The listing builds one solid part. Answer for the finished solid, in the listing's coordinates (mm). Coordinates: 2 decimals unless noted, no trailing zeros. Loops run counter-clockwise (first coordinate to the right, second up) from the corner with the lowest first, then second, coordinate; pieces in that order, holes last. Notation, with made-up numbers: (65, 80.25) -> (113, 80.25) arc R18 cw to (113, 112.25) -> close; hole circle Ø8 at (42.5, 20). An arc over 180 degrees is marked (long way). Answer in a Markdown table with one row per item.
```python
from build123d import *

# Parameters (mm, degrees)
SKETCH1_R           = 8
BOSS_EXTRUDE1_DEPTH = 3
CUT_EXTRUDE1_DEPTH  = 133.578278764
CUT_EXTRUDE8_DEPTH  = 10
FILLET2_R           = 5
FILLET3_R           = 5
FILLET4_R           = 5


with BuildPart() as part:
    # Sketch1 → Boss-Extrude1 (new body)
    with BuildSketch(Plane.XY):
        with BuildLine():
            Line((0, -12), (-120, -12))
            ThreePointArc((-120, -12), (-132, 0), (-120, 12))
            Line((-120, 12), (0, 12))
            ThreePointArc((0, 12), (12, 0), (0, -12))
        make_face()
        with Locations((-120, 0)):
            Circle(SKETCH1_R, mode=Mode.SUBTRACT)
        with Locations(Location((0, 0, 0), (0, 0, 180))):
            Circle(SKETCH1_R, mode=Mode.SUBTRACT)
    extrude(amount=BOSS_EXTRUDE1_DEPTH)

    # Sketch2 → Cut-Extrude1 (cut, through all)
    with BuildSketch(Plane.XY.offset(3)):
        with BuildLine():
            Line((-17.036725037, 6), (-20.036725037, 6))
            ThreePointArc((-20.036725037, 6), (-18.824439071, 9.116514898), (-17.130976336, 12))
            Line((-17.130976336, 12), (-13.5, 12))
            ThreePointArc((-13.5, 12), (-15.560298648, 9.172082969), (-17.036725037, 6))
        make_face()
        with BuildLine():
            Line((-102.963274963, 6), (-99.963274963, 6))
            ThreePointArc((-99.963274963, 6), (-101.175560929, 9.116514898), (-102.869023664, 12))
            Line((-102.869023664, 12), (-106.5, 12))
            ThreePointArc((-106.5, 12), (-104.439701352, 9.172082969), (-102.963274963, 6))
        make_face()
    extrude(amount=-CUT_EXTRUDE1_DEPTH, mode=Mode.SUBTRACT)

    # Sketch5 → Cut-Extrude8 (cut)
    with BuildSketch(Plane.XY.offset(3)):
        with BuildLine():
            Line((-1.731193523, -11.858337769), (-1.731193523, -12))
            Line((-1.731193523, -12), (-22.731193523, -12))
            Line((-22.731193523, -12), (-22.731193523, -2.344249067))
            Line((-22.731193523, -2.344249067), (-22.731193523, -1.572214532))
            Line((-22.731193523, -1.572214532), (-11.880460729, -1.572214532))
            ThreePointArc((-11.880460729, -1.572214532), (-8.530554828, -8.417056492), (-1.731193523, -11.858337769))
        make_face()
    extrude(amount=-CUT_EXTRUDE8_DEPTH, mode=Mode.SUBTRACT)

    # Fillet2
    fillet2_edges = [part.edges().sort_by_distance(p)[0] for p in [
        (-22.731193523, -1.572214532, 1.5),
    ]]
    fillet(fillet2_edges, radius=FILLET2_R)

    # Fillet3
    fillet3_edges = [part.edges().sort_by_distance(p)[0] for p in [
        (-11.880460729, -1.572214532, 1.5),
    ]]
    fillet(fillet3_edges, radius=FILLET3_R)

    # Fillet4
    fillet4_edges = [part.edges().sort_by_distance(p)[0] for p in [
        (-22.731193523, -12, 1.5),
    ]]
    fillet(fillet4_edges, radius=FILLET4_R)


solid = part.part
```
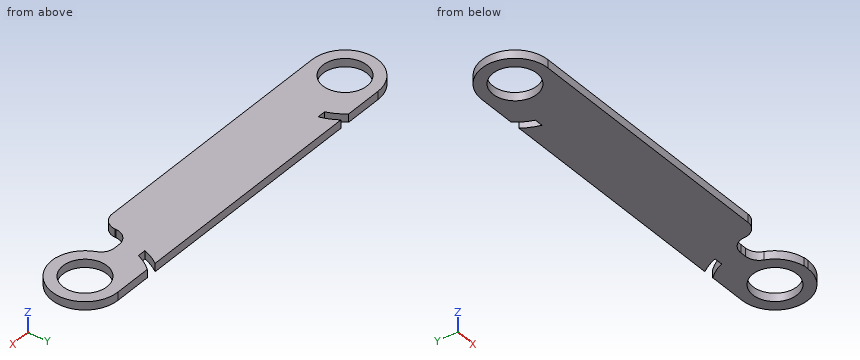
Item 1: Find the intervals of material crossed by probe 1 along Y at (x, z) = (-120, 1.75); probe 2 along X at (y, z) = (1, 0.35); probe 3 along X at (y, z) = (11, 0.7), in increasing order.
Findings below:
| item | result |
|---|---|
| probe 1 | y = -12 to -8, 8 to 12 |
| probe 2 | x = -131.96 to -127.94, -112.06 to -7.94, 7.94 to 11.96 |
| probe 3 | x = -124.8 to -105.67, -102.21 to -17.79, -14.33 to 4.8 |
Item 2: A cutting plane is placed at B-B, the plane x = 2.5. Determine the outline of the cut face in (y, z).
Findings below:
| item | result |
|---|---|
| outline | (-11.74, 0) -> (-7.6, 0) -> (-7.6, 3) -> (-11.74, 3) -> close; (7.6, 0) -> (11.74, 0) -> (11.74, 3) -> (7.6, 3) -> close |
Item 3: A cutting plane is placed at A-A, the plane z = 1.5. Determine the outline of the cut face in (x, y), plus the area to 3 significant figures.
Findings below:
| item | result |
|---|---|
| outline | (-120, -12) -> (-27.73, -12) arc R5 ccw to (-22.73, -7) -> (-22.73, -6.57) arc R5 cw to (-17.73, -1.57) -> (-15.66, -1.57) arc R5 cw to (-11.05, -4.64) arc R11.98 ccw to (-1.73, -11.86) -> (-1.73, -12) -> (0, -12) arc R12 ccw to (0, 12) -> (-13.5, 12) arc R18.06 ccw to (-17.04, 6) -> (-20.04, 6) arc R20.92 cw to (-17.13, 12) -> (-102.87, 12) arc R20.92 cw to (-99.96, 6) -> (-102.96, 6) arc R18.06 ccw to (-106.5, 12) -> (-120, 12) arc R12 ccw to start; hole circle Ø16 at (-120, 0); hole circle Ø16 at (0, 0) |
| area | 2,750 mm2 |
Item 4: Flat-ended cylindrical pins translate along their axes: pin 1 Ø13 at (x, y) = (0, 0) entering from +Z; pin 2 Ø0.5 at (y, z) = (-6.5, 2) entering from +X. Find the tip coordinate at first contact, or state that the pin passes through.
Findings below:
| item | result |
|---|---|
| pin 1 | passes through |
| pin 2 | stops at x = 10.24 |
Item 5: A cutting plane is placed at C-C, the plane y = -10. Determine the outline of the cut face in (x, z), plus the area to 3 significant figures.
Findings below:
| item | result |
|---|---|
| outline | (-126.63, 0) -> (-23.73, 0) -> (-23.73, 3) -> (-126.63, 3) -> close; (-6.6, 0) -> (6.63, 0) -> (6.63, 3) -> (-6.6, 3) -> close |
| area | 348 mm2 |
Item 6: A cutting plane is placed at D-D, the plane y = 4. Determine the outline of the cut face in (x, z), plus the area to 3 significant figures.
Findings below:
| item | result |
|---|---|
| outline | (-131.31, 0) -> (-126.93, 0) -> (-126.93, 3) -> (-131.31, 3) -> close; (-113.07, 0) -> (-6.93, 0) -> (-6.93, 3) -> (-113.07, 3) -> close; (6.93, 0) -> (11.31, 0) -> (11.31, 3) -> (6.93, 3) -> close |
| area | 345 mm2 |
